Read the model definition and answer for the solid it produces. Units are mm, in the model's axes. A direction names the side the tool comes from. Coordinates: 2 decimals unless noted, no trailing zeros. Write each loop counter-clockwise with the first axis right and the second up, starting at its lowest first coordinate (ties: lowest second). Pieces come first, ordered by that corner, then holes. Notation, with made-up numbers: (67.5, -17.5) -> (83.5, -17.5) arc R32 cw to (83.5, 11.5) -> close; hole circle Ø4 at (8, 22). An arc over 180 degrees is marked (long way). Write item = value, one per line. Start each with the question number.
1) Section D-D (z = -50) is taken. Determine the outline of the cut face in (x, y).
2) Section A-A (x = 0) is taken. Determine the outline of the cut face in (y, z), plus the area to 3 significant figures.
3) Section C-C (y = 4.25) is taken. Determine the outline of the cut face in (x, z), plus the area to 3 significant figures.
4) Flat-ended cylindrical pins translate along their axes: pin 1 Ø3 at (x, y) = (-64, 4.5) entering from -Z; pin 2 Ø4 at (y, z) = (9, -33.5) entering from +X; pin 3 Ø9 at (x, z) = (0, 0) entering from -Y; pin 4 Ø1 at (y, z) = (1.5, 58) entering from +X. Find the tip coordinate at first contact, or state that the pin passes through.
5) For a pull along Z with two mould halves and no side action, classify faces 3 (the face through (41.53, 4.93, 79.845)), 4 (the face through (-1.08, 4.93, -4.88)), 5 (the face through (19, 0, -1)), 6 (the face through (65, 5, 35)) as released by +Z, released by -Z, zero draft, split by the parting line, or undercut.
6) Section B-B (z = 0) is taken. Determine the outline of the cut face in (x, y).
7) A tool of negligible diameter and unlimited length cuts with its end or side. For faces 1 (the face through (-65, 5, 35)), 2 (the face through (19, 10, -1)), from which of +Z, -Z, +X, -X, +Y, -Y can it reach the whole face along a straight path? Write none if from no direction.
8) Find the intervals of material crossed by line 1 along Z through (x, y) = (0, 7.25); line 2 along X through (y, z) = (0.5, -29); line 3 along X through (y, z) = (7, 11.5), in increasing order. Write a range as from..to.
from build123d import *

# Parameters (mm, degrees)
SKETCH1_R           = 90
SKETCH1_W           = 13
SKETCH1_H           = 70
BOSS_EXTRUDE1_DEPTH = 10
CUT_EXTRUDE1_REACH  = 12
SKETCH2_R           = 5


with BuildPart() as part:
    # Sketch1 → Boss-Extrude1 (new body)
    with BuildSketch(Plane(origin=(0, 0, 0), x_dir=(1, 0, 0), z_dir=(0, 1, 0))):
        Circle(SKETCH1_R)
        with Locations((-65, 0)):
            Rectangle(SKETCH1_W, SKETCH1_H, mode=Mode.SUBTRACT)
        with Locations((65, 0)):
            Rectangle(SKETCH1_W, SKETCH1_H, mode=Mode.SUBTRACT)
    extrude(amount=BOSS_EXTRUDE1_DEPTH)

    # Sketch2 → Cut-Extrude1 (cut, up to next)
    with BuildSketch(Plane.XZ, mode=Mode.PRIVATE) as cut_extrude1_sk1:
        Circle(SKETCH2_R)
    cut_extrude1_tool1 = extrude(cut_extrude1_sk1.sketch, amount=-CUT_EXTRUDE1_REACH, mode=Mode.PRIVATE) & part.part
    add(cut_extrude1_tool1.solids().sort_by_distance((0, 0, 0))[0], mode=Mode.SUBTRACT)


solid = part.part
Answer key:
q1.outline = (-74.83, 0) -> (74.83, 0) -> (74.83, 10) -> (-74.83, 10) -> close
q2.outline = (0, -90) -> (10, -90) -> (10, -5) -> (0, -5) -> close; (0, 5) -> (10, 5) -> (10, 90) -> (0, 90) -> close
q2.area = 1,700 mm^2
q3.outline = circle Ø180 at (0, 0); hole (-71.5, -35) -> (-58.5, -35) -> (-58.5, 35) -> (-71.5, 35) -> close; hole circle Ø10 at (0, 0); hole (58.5, -35) -> (71.5, -35) -> (71.5, 35) -> (58.5, 35) -> close
q3.area = 23,500 mm^2
q4.pin_1 = -64.76
q4.pin_2 = 84.31
q4.pin_3 = through
q4.pin_4 = 69.24
q5.face_3 = split by the parting line
q5.face_4 = undercut
q5.face_5 = zero draft
q5.face_6 = undercut
q6.outline = (-90, 0) -> (-71.5, 0) -> (-71.5, 10) -> (-90, 10) -> close; (-58.5, 0) -> (-5, 0) -> (-5, 10) -> (-58.5, 10) -> close; (5, 0) -> (58.5, 0) -> (58.5, 10) -> (5, 10) -> close; (71.5, 0) -> (90, 0) -> (90, 10) -> (71.5, 10) -> close
q7.face_1 = +Y, -Y
q7.face_2 = +Z, -Z, +X, -X, +Y
q8.line_1 = -90..-5, 5..90
q8.line_2 = -85.2..-71.5, -58.5..58.5, 71.5..85.2
q8.line_3 = -89.26..-71.5, -58.5..58.5, 71.5..89.26
